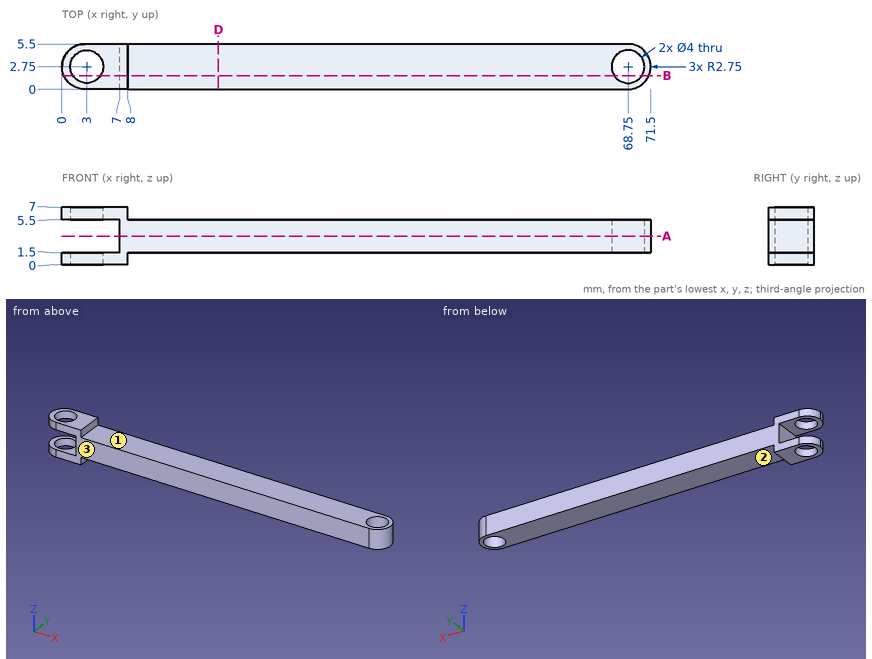
Design review of the part shown in the three views and the two pictorial views. Dimensions are in mm from the part's minimum x, y and z. A direction names the side the tool comes from. Coordinates: 2 decimals unless noted, no trailing zeros. Write each loop counter-clockwise with the first axis right and the second up, starting at its lowest first coordinate (ties: lowest second). Pieces come first, ordered by that corner, then holes.
1) Machinability: for the marked faces 1, 2 and 3, which of the approach directions +Z, -Z, +X, -X, +Y, -Y give a long, thin tool a straight path to every point of the face, cutting with its end or side? Answer none if there is none.
2) We need section A-A on z = 3.5. State the section outline as (x, y) points, then the cut area to 3 significant figures.
3) We need section B-B on y = 1.65. State the section outline as (x, z) points.
4) To check wall thickness, follow probe 1 along Z at (x, y) = (5, 0.35); probe 2 along Z at (x, y) = (20.5, 2); probe 3 along X at (y, z) = (2.7, 3.75). State the ranges of each line that lie inside material, in increasing order.
5) We need section D-D on x = 19. State the section outline as (y, z) points, then the cut area to 3 significant figures.
6) Clearance check with flat-ended pins moving along their axes: pin 1 Ø2 at (y, z) = (4.5, 4.5) entering from +X; pin 2 Ø1.6 at (y, z) = (3.5, 6.5) entering from +X; pin 3 Ø3 at (x, y) = (56, 3) entering from -Z. State where each tip first meets the part, or that it passes through.
Answer list:
1. face 1: +Z, +X, +Y, -Y
1. face 2: -Z, +X, +Y, -Y
1. face 3: +Z, -Z, +X, -X, -Y
2. outline: (7, 0) - (68.75, 0) arc R2.75 ccw to (68.75, 5.5) - (7, 5.5) - close; hole circle Ø4 at (68.75, 2.75)
2. area: 339 mm2
3. outline: (0.23, 0) - (1.33, 0) - (1.33, 1.5) - (0.23, 1.5) - close; (0.23, 5.5) - (1.33, 5.5) - (1.33, 7) - (0.23, 7) - close; (4.67, 0) - (8, 0) - (8, 1.5) - (67.08, 1.5) - (67.08, 5.5) - (8, 5.5) - (8, 7) - (4.67, 7) - (4.67, 5.5) - (7, 5.5) - (7, 1.5) - (4.67, 1.5) - close; (70.42, 1.5) - (71.27, 1.5) - (71.27, 5.5) - (70.42, 5.5) - close
4. probe 1: z = 0 to 1.5, 5.5 to 7
4. probe 2: z = 1.5 to 5.5
4. probe 3: x = 7 to 66.75, 70.75 to 71.5
5. outline: (0, 1.5) - (5.5, 1.5) - (5.5, 5.5) - (0, 5.5) - close
5. area: 22.0 mm2
6. pin 1: stops at x = 71.4
6. pin 2: stops at x = 8
6. pin 3: stops at z = 1.5
